from build123d import *

# Parameters (mm, degrees)
F0_W     = 279.4
F0_H     = 101.6
F1_DEPTH = 12.7
F2_R     = 12.7
F3_R     = 6.35
F3_R_2   = 3.96875
F4_DEPTH = 22.86


with BuildPart() as f1:
    # F0 (on Front) → F1 (new body)
    with BuildSketch(Plane.XZ):
        with Locations((139.7, 50.8)):
            Rectangle(F0_W, F0_H)
    extrude(amount=F1_DEPTH)

    # F2
    f2_edges = [f1.edges().sort_by_distance(p)[0] for p in [
        (0, -6.35, 101.6),
        (279.4, -6.35, 101.6),
        (279.4, -6.35, 0),
        (0, -6.35, 0),
    ]]
    fillet(f2_edges, radius=F2_R)

    # F3 (on Front) → F4 (cut)
    with BuildSketch(Plane.XZ):
        with Locations((15.989296, 50.838098)):
            Circle(F3_R)
        with Locations((41.200113, 50.979976)):
            Circle(F3_R_2)
        with Locations((130.282387, 51.25564)):
            Circle(F3_R_2)
        with Locations((266.039491, 50.202426)):
            Circle(F3_R)
    extrude(amount=F4_DEPTH, mode=Mode.SUBTRACT)


solid = f1.part
Work out the finished part from the listing and answer in its coordinate system (mm). Round coordinates to 2 decimals unless told otherwise and drop trailing zeros. Write each loop counter-clockwise with the first axis right and the second up, starting at its lowest first coordinate (ties: lowest second). Pieces come first, ordered by that corner, then holes.
1) Straight lines are drawn through the part: line 1 (X direction, y = -2.75, z = 45); line 2 (X direction, y = -5.25, z = 49); line 3 (X direction, y = -7.75, z = 90). For each, find the intervals that lie inside material, in ascending order.
2) Given pin 1 Ø10 at (x, z) = (266.04, 50.2) entering from +Y; pin 2 Ø3 at (y, z) = (-9.5, 10.5) entering from -X, each flat-ended and moving along its own axis, determine where each tip first touches the part or whether it passes through.
3) A cutting plane is placed at A-A (y = -3.75). Give the vertices of the cut face in (x, z).
4) The mould has two halves that part along Z. Classify faces 1 (the cylindrical face through (275.78, -6.44, 97.78)), 2 (the flat face through (138, -12.7, 52)), 3 (the cylindrical face through (3.62, -6.44, 3.82)), 4 (the cylindrical face through (19.403, -6.261, 56.192)): pulls with the +Z half, pulls with the -Z half, needs draft (parallel to the pull), parting line crosses it, or undercut.
Completed:
1. line 1: x = 0 to 13.49, 18.49 to 262.4, 269.68 to 279.4
1. line 2: x = 0 to 9.91, 22.07 to 37.76, 44.64 to 127.02, 133.55 to 259.8, 272.27 to 279.4
1. line 3: x = 0.05 to 279.35
2. pin 1: passes through
2. pin 2: stops at x = 0.02
3. outline: (0, 12.7) arc R12.7 ccw to (12.7, 0) - (266.7, 0) arc R12.7 ccw to (279.4, 12.7) - (279.4, 88.9) arc R12.7 ccw to (266.7, 101.6) - (12.7, 101.6) arc R12.7 ccw to (0, 88.9) - close; hole circle Ø12.7 at (15.99, 50.84); hole circle Ø7.94 at (41.2, 50.98); hole circle Ø7.94 at (130.28, 51.26); hole circle Ø12.7 at (266.04, 50.2)
4. face 1: pulls with the +Z half
4. face 2: needs draft
4. face 3: pulls with the -Z half
4. face 4: undercut
